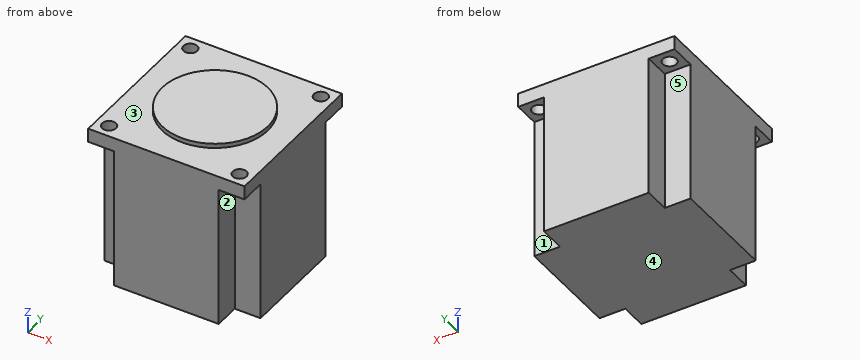
```python
from build123d import *

# Parameters (mm, degrees)
BOSS_EXTRUDE2_DEPTH = 51
SKETCH3_W           = 56.4
SKETCH3_H           = 56.4
SKETCH3_R           = 2.5
BOSS_EXTRUDE3_DEPTH = 5
SKETCH4_R           = 19.05
BOSS_EXTRUDE4_DEPTH = 1.6


with BuildPart() as part:
    # Sketch2 → Boss-Extrude2 (new body)
    with BuildSketch(Plane.XY):
        Polygon((-18.9, 28.2), (18.9, 28.2), (18.9, 18.9), (28.2, 18.9), (28.2, -18.9), (18.9, -18.9), (18.9, -28.2), (-18.9, -28.2), (-18.9, -18.9), (-28.2, -18.9), (-28.2, 18.9), (-18.9, 18.9), align=None)
    extrude(amount=BOSS_EXTRUDE2_DEPTH)

    # Sketch3 → Boss-Extrude3 (add)
    with BuildSketch(Plane.XY.offset(51)):
        Rectangle(SKETCH3_W, SKETCH3_H)
        with Locations((-23.55, 23.55)):
            Circle(SKETCH3_R, mode=Mode.SUBTRACT)
        with Locations((23.55, 23.55)):
            Circle(SKETCH3_R, mode=Mode.SUBTRACT)
        with Locations((23.55, -23.55)):
            Circle(SKETCH3_R, mode=Mode.SUBTRACT)
        with Locations((-23.55, -23.55)):
            Circle(SKETCH3_R, mode=Mode.SUBTRACT)
    extrude(amount=BOSS_EXTRUDE3_DEPTH)

    # Sketch4 → Boss-Extrude4 (add)
    with BuildSketch(Plane.XY.offset(56)):
        with Locations(Location((0, 0, 0), (0, 0, 180))):
            Circle(SKETCH4_R)
    extrude(amount=BOSS_EXTRUDE4_DEPTH)


solid = part.part
```
Here's how the part is built. I have some questions about the finished solid (model axes, mm). Face numbers are marked on the shaded views. A direction names the side the tool comes from. Coordinates: 2 decimals unless noted, no trailing zeros. Loops run counter-clockwise (first coordinate to the right, second up) from the corner with the lowest first, then second, coordinate; pieces in that order, holes last. Notation, with made-up numbers: (-30, -21) - (11, -21) arc R18 ccw to (11, 1) - close; hole circle Ø7 at (27, 7). An arc over 180 degrees is marked (long way). Answer as CSV lines item,"result".
Q1. If I drill on L1, parallel to Y at x = 23.55, z = 53.7; L2, parallel to Z at x = 5.5, y = -22.5; L3, parallel to X at y = 23, z = 53, over which ranges is the centre line in solid material (lowest first)? Write a range as [from, to].
Response:
L1,"[-28.2, -26.05], [-21.05, 21.05], [26.05, 28.2]"
L2,"[0, 56]"
L3,"[-28.2, -25.99], [-21.11, 21.11], [25.99, 28.2]"
Q2. If we section it at D-D, the plane y = 20: Write out the boundary of the cut face in (x, z).
Response:
outline,"(-28.2, 51) - (-18.9, 51) - (-18.9, 0) - (18.9, 0) - (18.9, 51) - (28.2, 51) - (28.2, 56) - (-28.2, 56) - close"
Q3. For the marked faces 1, 2, 3, 4 and 5, which set-ups out of +Z, -Z, +X, -X, +Y, -Y let a thin tool reach every point of the face, with its end or its side?
Response:
face 1,"-Z, +X, +Y"
face 2,"-Z, +X, -Y"
face 3,"+Z"
face 4,"-Z, +X, -X, +Y, -Y"
face 5,"-Z, -X, +Y"
Q4. For pin 1 (4 mm diameter, centred on x = 23.55, y = 23.55, fed in from +Z); pin 2 (3 mm diameter, centred on x = 22, z = 20.5, fed in from -Y); pin 3 (4.5 mm diameter, centred on x = -25.5, y = -23, fed in from -Z); pin 4 (3 mm diameter, centred on x = 21.5, z = 20.5, fed in from +Y), each with a flat end and sliding along its axis, tell me the tip position at first contact or that it passes through.
Response:
pin 1,"through"
pin 2,"y = -18.9"
pin 3,"z = 51"
pin 4,"y = 18.9"
Q5. If we section it at A-A, the plane y = -23.55: Write out the boundary of the cut face in (x, z), and give its area (3 significant figures).
Response:
outline,"(-28.2, 51) - (-26.05, 51) - (-26.05, 56) - (-28.2, 56) - close; (-21.05, 51) - (-18.9, 51) - (-18.9, 0) - (18.9, 0) - (18.9, 51) - (21.05, 51) - (21.05, 56) - (-21.05, 56) - close; (26.05, 51) - (28.2, 51) - (28.2, 56) - (26.05, 56) - close"
area,"2,160 mm2"
Q6. If we section it at C-C, the plane z = 34: Write out the boundary of the cut face in (x, y), and give its area (4 significant figures).
Response:
outline,"(-28.2, -18.9) - (-18.9, -18.9) - (-18.9, -28.2) - (18.9, -28.2) - (18.9, -18.9) - (28.2, -18.9) - (28.2, 18.9) - (18.9, 18.9) - (18.9, 28.2) - (-18.9, 28.2) - (-18.9, 18.9) - (-28.2, 18.9) - close"
area,"2,835 mm2"
